from build123d import *

# Parameters (mm, degrees)
F1_DEPTH = 714
F2_R     = 8
F3_DEPTH = 20
F2_R_2   = 12
F4_DEPTH = 15


with BuildPart() as f1:
    # F0 (on Front) → F1 (new body)
    with BuildSketch(Plane.XZ):
        Polygon((43.279102, 31.123051), (-96.720898, 31.123051), (-96.720898, 11.123051), (28.978059, 11.123051), (43.279102, 23.123051), align=None)
    extrude(amount=F1_DEPTH)

    # F2 (on face) → F3 (cut)
    with BuildSketch(Plane.XY.offset(31.123051)):
        with Locations((13.279102, -689)):
            Circle(F2_R)
        with Locations((-71.720898, -689)):
            Circle(F2_R)
        with Locations((-6.720898, -607)):
            Circle(F2_R)
        with Locations((13.279102, -525)):
            Circle(F2_R)
        with Locations((-71.720898, -525)):
            Circle(F2_R)
        with Locations((-6.720898, -443)):
            Circle(F2_R)
        with Locations((13.279102, -361)):
            Circle(F2_R)
        with Locations((-71.720898, -361)):
            Circle(F2_R)
        with Locations((-6.720898, -279)):
            Circle(F2_R)
        with Locations((13.279102, -197)):
            Circle(F2_R)
        with Locations((-71.720898, -197)):
            Circle(F2_R)
        with Locations((-6.720898, -115)):
            Circle(F2_R)
        with Locations((13.279102, -33)):
            Circle(F2_R)
        with Locations((-71.720898, -33)):
            Circle(F2_R)
    extrude(amount=-F3_DEPTH, mode=Mode.SUBTRACT)

    # F2 (on face) → F4 (cut)
    with BuildSketch(Plane.XY.offset(31.123051)):
        with Locations((-71.720898, -689)):
            Circle(F2_R_2)
        with Locations((-71.720898, -689)):
            Circle(F2_R, mode=Mode.SUBTRACT)
        with Locations((13.279102, -689)):
            Circle(F2_R_2)
        with Locations((13.279102, -689)):
            Circle(F2_R, mode=Mode.SUBTRACT)
        with Locations((-6.720898, -607)):
            Circle(F2_R_2)
        with Locations((-6.720898, -607)):
            Circle(F2_R, mode=Mode.SUBTRACT)
        with Locations((13.279102, -525)):
            Circle(F2_R_2)
        with Locations((13.279102, -525)):
            Circle(F2_R, mode=Mode.SUBTRACT)
        with Locations((-71.720898, -525)):
            Circle(F2_R_2)
        with Locations((-71.720898, -525)):
            Circle(F2_R, mode=Mode.SUBTRACT)
        with Locations((-6.720898, -443)):
            Circle(F2_R_2)
        with Locations((-6.720898, -443)):
            Circle(F2_R, mode=Mode.SUBTRACT)
        with Locations((13.279102, -361)):
            Circle(F2_R_2)
        with Locations((13.279102, -361)):
            Circle(F2_R, mode=Mode.SUBTRACT)
        with Locations((-71.720898, -361)):
            Circle(F2_R_2)
        with Locations((-71.720898, -361)):
            Circle(F2_R, mode=Mode.SUBTRACT)
        with Locations((-6.720898, -279)):
            Circle(F2_R_2)
        with Locations((-6.720898, -279)):
            Circle(F2_R, mode=Mode.SUBTRACT)
        with Locations((13.279102, -197)):
            Circle(F2_R_2)
        with Locations((13.279102, -197)):
            Circle(F2_R, mode=Mode.SUBTRACT)
        with Locations((-71.720898, -197)):
            Circle(F2_R_2)
        with Locations((-71.720898, -197)):
            Circle(F2_R, mode=Mode.SUBTRACT)
        with Locations((-6.720898, -115)):
            Circle(F2_R_2)
        with Locations((-6.720898, -115)):
            Circle(F2_R, mode=Mode.SUBTRACT)
        with Locations((13.279102, -33)):
            Circle(F2_R_2)
        with Locations((13.279102, -33)):
            Circle(F2_R, mode=Mode.SUBTRACT)
        with Locations((-71.720898, -33)):
            Circle(F2_R_2)
        with Locations((-71.720898, -33)):
            Circle(F2_R, mode=Mode.SUBTRACT)
    extrude(amount=-F4_DEPTH, mode=Mode.SUBTRACT)


solid = f1.part
Could you check a few things on this model? Use its own coordinates, in mm. A direction names the side the tool comes from. Coordinates: 2 decimals unless noted, no trailing zeros. Write each loop counter-clockwise with the first axis right and the second up, starting at its lowest first coordinate (ties: lowest second). Pieces come first, ordered by that corner, then holes. Notation, with made-up numbers: M 47,-18 L 78,-18 A16 ccw 78,4 Z; hole C 83.5,30.5 d5. An arc over 180 degrees is marked long. One line per question, with ' | ' between items.
1) Imagine slicing it at C-C, the plane y = -115. Write out the boundary of the cut face in (x, z), and give its area (3 significant figures).
Checks:
outline: M -96.72,11.12 L -14.72,11.12 L -14.72,16.12 L -18.72,16.12 L -18.72,31.12 L -96.72,31.12 Z; M 1.28,11.12 L 28.98,11.12 L 43.28,23.12 L 43.28,31.12 L 5.28,31.12 L 5.28,16.12 L 1.28,16.12 Z | area: 2,270 mm²
2) I need wall thicknesses on probe 1 along X at (y, z) = (-689, 21.25); probe 2 along X at (y, z) = (-525, 14.5); probe 3 along Y at (x, z) = (11, 15.5). Which ranges of each line are inside material? Lowest first, please. Write a range as [from, to].
Checks:
probe 1: [-96.72, -83.72], [-59.72, 1.28], [25.28, 41.05] | probe 2: [-96.72, -79.72], [-63.72, 5.28], [21.28, 33] | probe 3: [-714, -696.67], [-681.33, -532.67], [-517.33, -368.67], [-353.33, -204.67], [-189.33, -40.67], [-25.33, 0]
3) Imagine slicing it at B-B, the plane z = 26.25. Give the number of separate pieces and of enclosed holes in the cut face, and give its area (3 significant figures).
Checks:
separate pieces: 1 | enclosed holes: 14 | area: 93,600 mm²
4) If we mould it in two halves opening along X, with no side actions, what happens to faces 3 (the face through (-26, -352, 31.123)), 4 (the face through (-68.029, -532.097, 13.658)), 5 (the face through (21.1, -527.5, 16.123))? For each: released by +X, released by -X, zero draft, split by the parting line, or undercut.
Checks:
face 3: zero draft | face 4: undercut | face 5: undercut
5) For pin 1 Ø12 at (x, y) = (-76.5, -691) entering from +Z; pin 2 Ø13 at (x, y) = (-71.72, -33) entering from -Z, each with a flat end and sliding along its axis, tell me the tip position at first contact or that it passes through.
Checks:
pin 1: z = 16.12 | pin 2: through
6) Imagine slicing it at D-D, the plane y = -310.5. Write out the boundary of the cut face in (x, z), and give its area (3 significant figures).
Checks:
outline: M -96.72,11.12 L 28.98,11.12 L 43.28,23.12 L 43.28,31.12 L -96.72,31.12 Z | area: 2,710 mm²
7) For faces 1 (the face through (11.5, -204.8, 13.7)), 2 (the face through (-73.28, -677.1, 23.73)), which set-ups out of +Z, -Z, +X, -X, +Y, -Y let a thin tool reach every point of the face, with its end or its side?
Checks:
face 1: +Z, -Z | face 2: +Z
8) Imagine slicing it at A-A, the plane y = -197. Write out the boundary of the cut face in (x, z).
Checks:
outline: M -96.72,11.12 L -79.72,11.12 L -79.72,16.12 L -83.72,16.12 L -83.72,31.12 L -96.72,31.12 Z; M -63.72,11.12 L 5.28,11.12 L 5.28,16.12 L 1.28,16.12 L 1.28,31.12 L -59.72,31.12 L -59.72,16.12 L -63.72,16.12 Z; M 21.28,11.12 L 28.98,11.12 L 43.28,23.12 L 43.28,31.12 L 25.28,31.12 L 25.28,16.12 L 21.28,16.12 Z
